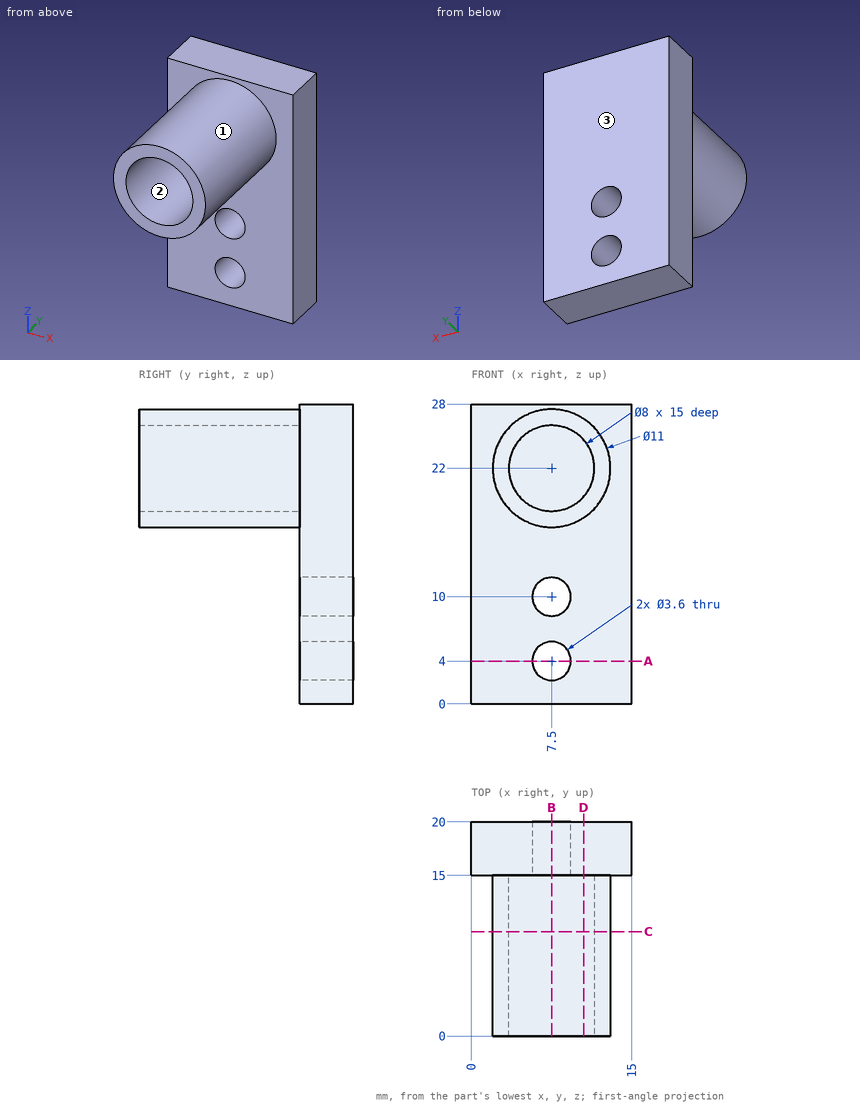
Answer from the drawing. Dimensions are ordinates in mm from the lowest x, y and z of the part. Coordinates: 2 decimals unless noted, no trailing zeros. Loops run counter-clockwise (first coordinate to the right, second up) from the corner with the lowest first, then second, coordinate; pieces in that order, holes last. Notation, with made-up numbers: (-20, 19) - (12, 19) arc R6 ccw to (12, 29) - close; hole circle Ø8 at (-38, -39). An arc over 180 degrees is marked (long way). Answer in a Markdown table with one row per item.
1. Given pin 1 (7.5 mm diameter, centred on x = 8.5, z = 11, fed in from -Y); pin 2 (2 mm diameter, centred on x = 5.5, y = 8, fed in from -Z); pin 3 (8 mm diameter, centred on x = 2.5, y = 3, fed in from +Z); pin 4 (2 mm diameter, centred on x = 7.5, z = 4, fed in from +Y), each flat-ended and moving along its own axis, determine where each tip first touches the part or whether it passes through.
Conclusion:
| item | result |
|---|---|
| pin 1 | stops at y = 15 |
| pin 2 | stops at z = 16.59 |
| pin 3 | stops at z = 27.41 |
| pin 4 | passes through |
2. Determine the mould class of the marked faces 1, 2 and 3 for opening direction X: +X half, -X half, draft (parallel to the pull), parting line (faces both ways), or undercut.
Conclusion:
| item | result |
|---|---|
| face 1 | parting line |
| face 2 | undercut |
| face 3 | draft |
3. Find section A-A, the plane z = 4. Write down the section's boundary in (x, y), then the cut area to 3 significant figures.
Conclusion:
| item | result |
|---|---|
| outline | (0, 15) - (5.7, 15) - (5.7, 20) - (0, 20) - close; (9.3, 15) - (15, 15) - (15, 20) - (9.3, 20) - close |
| area | 57.0 mm² |
4. Find section D-D, the plane x = 10.5. Write down the section's boundary in (y, z).
Conclusion:
| item | result |
|---|---|
| outline | (0, 17.39) - (15, 17.39) - (15, 0) - (20, 0) - (20, 28) - (15, 28) - (15, 26.61) - (0, 26.61) - (0, 24.65) - (15, 24.65) - (15, 19.35) - (0, 19.35) - close |
5. Find section B-B, the plane x = 7.5. Write down the section's boundary in (y, z).
Conclusion:
| item | result |
|---|---|
| outline | (0, 16.5) - (15, 16.5) - (15, 11.8) - (20, 11.8) - (20, 28) - (15, 28) - (15, 27.5) - (0, 27.5) - (0, 26) - (15, 26) - (15, 18) - (0, 18) - close; (15, 0) - (20, 0) - (20, 2.2) - (15, 2.2) - close; (15, 5.8) - (20, 5.8) - (20, 8.2) - (15, 8.2) - close |
6. Find section C-C, the plane y = 9.75. Write down the section's boundary in (x, z), then the cut area to 3 significant figures.
Conclusion:
| item | result |
|---|---|
| outline | circle Ø11 at (7.5, 22); hole circle Ø8 at (7.5, 22) |
| area | 44.8 mm² |
7. Straight lines are drawn through the part: line 1 (Z direction, x = 7.5, y = 5.5); line 2 (Z direction, x = 7.5, y = 16.15); line 3 (Y direction, x = 10.5, z = 7.5). For each, find the intervals that lie inside material, in ascending order.
Conclusion:
| item | result |
|---|---|
| line 1 | z = 16.5 to 18, 26 to 27.5 |
| line 2 | z = 0 to 2.2, 5.8 to 8.2, 11.8 to 28 |
| line 3 | y = 15 to 20 |
